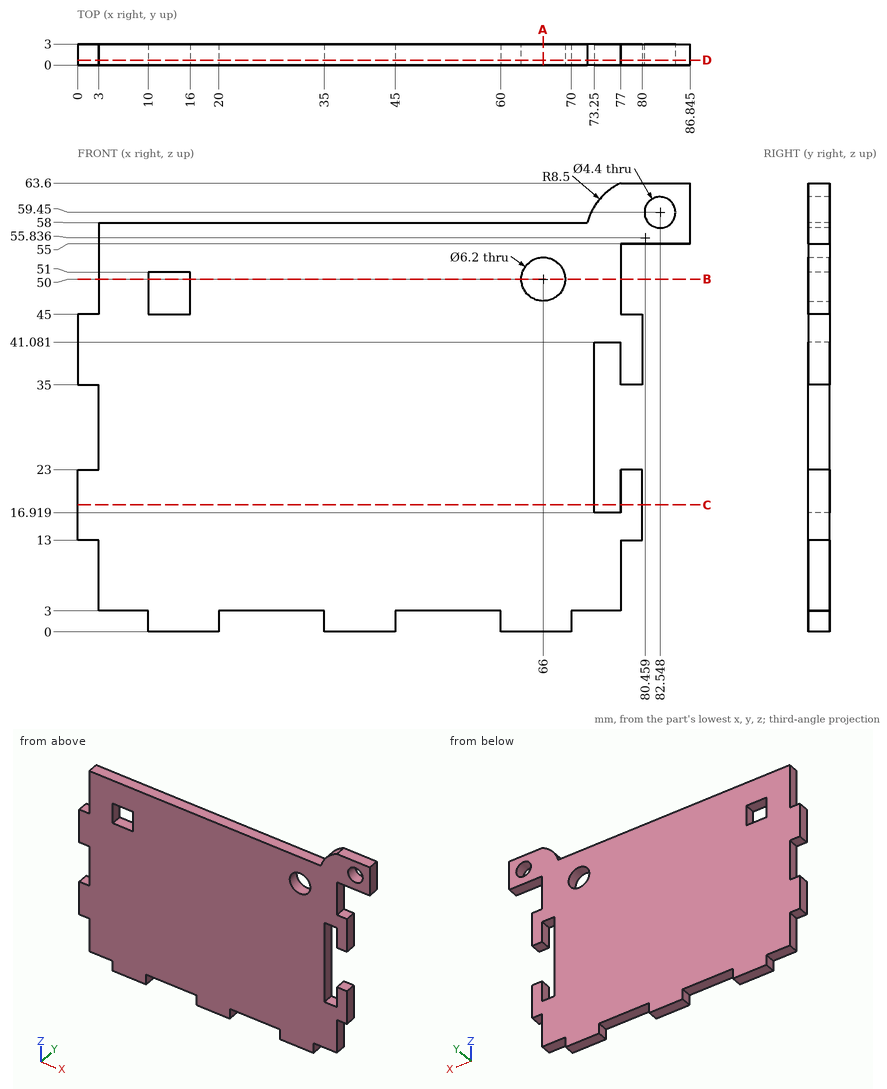
Could you check a few things on this drawing? It's one solid part, dimensions in mm from its lowest x, y, z. Give positions to 0.01 mm unless a question says otherwise; leave off trailing zeros. Order: outer loops, then holes, each group sorted by start corner. A loop starts at its lowest first (then second) coordinate and runs counter-clockwise, first axis right, second up.
1. Suppose I cut it at C-C (z = 18). Write out the boundary of the cut face in (x, y), plus the area to 3 significant figures.
Answers below:
outline: (0, 0) - (73.25, 0) - (73.25, 3) - (0, 3) - close; (77, 0) - (80, 0) - (80, 3) - (77, 3) - close
area: 229 mm2
2. Suppose I cut it at D-D (y = 0.7). State how many separate pieces and enclosed holes the cut face has, plus the area to 3 significant figures.
Answers below:
separate pieces: 1
enclosed holes: 3
area: 4,210 mm2
3. For pin 1 (1.5 mm diameter, centred on y = 2, z = 28.5, fed in from +X); pin 2 (0.9 mm diameter, centred on x = 52, y = 1, fed in from -Z); pin 3 (1.5 mm diameter, centred on y = 0.5, z = 26, fed in from -X); pin 4 (8 mm diameter, centred on x = 77.5, z = 24.5, fed in from -Y), each with a flat end and sliding along its axis, tell me the tip position at first contact or that it passes through.
Answers below:
pin 1: stops at x = 73.25
pin 2: stops at z = 3
pin 3: stops at x = 3
pin 4: stops at y = 0
4. I need wall thicknesses on L1, parallel to X at y = 1, z = 50; L2, parallel to Z at x = 66, y = 1.9; L3, parallel to X at y = 2, z = 40.5. Which ranges of each line are inside material? Lowest first, please.
Answers below:
L1: x = 3 to 10, 16 to 62.9, 69.1 to 77
L2: z = 0 to 46.9, 53.1 to 58
L3: x = 0 to 73.25, 77 to 80
5. Suppose I cut it at A-A (x = 66). Write out the boundary of the cut face in (y, z).
Answers below:
outline: (0, 0) - (3, 0) - (3, 46.9) - (0, 46.9) - close; (0, 53.1) - (3, 53.1) - (3, 58) - (0, 58) - close
6. Suppose I cut it at B-B (z = 50). Write out the boundary of the cut face in (x, y).
Answers below:
outline: (3, 0) - (10, 0) - (10, 3) - (3, 3) - close; (16, 0) - (62.9, 0) - (62.9, 3) - (16, 3) - close; (69.1, 0) - (77, 0) - (77, 3) - (69.1, 3) - close
